from build123d import *

# Parameters (mm, degrees)
SKETCH040_W     = 20
SKETCH040_H     = 8
PAD021_DEPTH    = 10
POCKET019_DEPTH = 20
SKETCH042_R     = 1.5
POCKET020_DEPTH = 4
SKETCH043_W     = 4
SKETCH043_H     = 4.5
POCKET021_DEPTH = 5


with BuildPart() as part:
    # Sketch040 → Pad021 (new body)
    with BuildSketch(Plane.XY):
        Rectangle(SKETCH040_W, SKETCH040_H)
    extrude(amount=PAD021_DEPTH)

    # Sketch041 (on Face2 of Pad021) → Pocket019 (cut)
    with BuildSketch(Plane.YZ.offset(10)):
        Polygon((-4, 6.5), (-2.5, 10), (1, 10), (4, 6.5), (5, 6.5), (5, 11), (-5, 11), (-5, 6.5), align=None)
    extrude(amount=-POCKET019_DEPTH, mode=Mode.SUBTRACT)

    # Sketch042 (on Face8 of Pocket019) → Pocket020 (cut)
    with BuildSketch(Plane.XY.offset(10)):
        with Locations((-7.5, -0.75)):
            Circle(SKETCH042_R)
        with Locations((-2.5, -0.75)):
            Circle(SKETCH042_R)
        with Locations((2.5, -0.75)):
            Circle(SKETCH042_R)
        with Locations((7.5, -0.75)):
            Circle(SKETCH042_R)
    extrude(amount=-POCKET020_DEPTH, mode=Mode.SUBTRACT)

    # Sketch043 (on Face6 of Pocket020) → Pocket021 (cut)
    with BuildSketch(Plane.XZ.offset(4)):
        with Locations((-7.5, 3.25)):
            Rectangle(SKETCH043_W, SKETCH043_H)
        with Locations((-2.5, 3.25)):
            Rectangle(SKETCH043_W, SKETCH043_H)
        with Locations((2.5, 3.25)):
            Rectangle(SKETCH043_W, SKETCH043_H)
        with Locations((7.5, 3.25)):
            Rectangle(SKETCH043_W, SKETCH043_H)
    extrude(amount=-POCKET021_DEPTH, mode=Mode.SUBTRACT)


solid = part.part
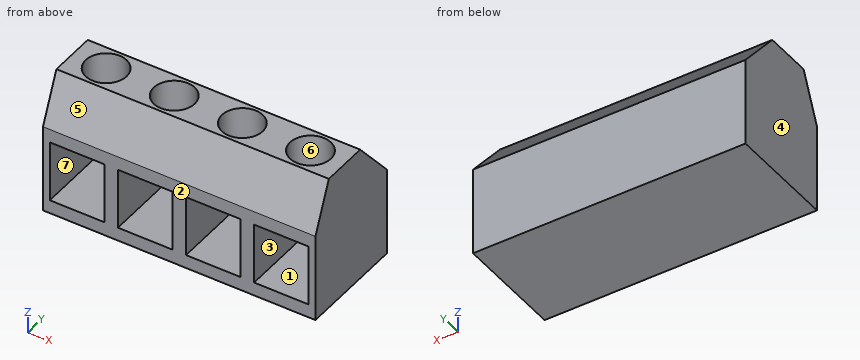
CAD build for the part. Positions are in the model's coordinates, mm. Face numbers are marked on the shaded views. A direction names the side the tool comes from. Give positions to 0.01 mm unless a question says otherwise; leave off trailing zeros. Loops run counter-clockwise (first coordinate to the right, second up) from the corner with the lowest first, then second, coordinate; pieces in that order, holes last. Notation, with made-up numbers: M 38.5,8.25 L 55.5,8.25 A16 cw 55.5,31.25 Z; hole C -19.75,22 d10. An arc over 180 degrees is marked long. Write each question's results on one line, items separated by ' | '.
Q1. Band-saw the part on C-C on y = -3. Write the cut outline in (x, z).
Geometry check:
outline: M -10,0 L 10,0 L 10,8.83 L -10,8.83 Z; hole M -9.5,1 L -5.5,1 L -5.5,5.5 L -9.5,5.5 Z; hole M -4.5,1 L -0.5,1 L -0.5,5.5 L -4.5,5.5 Z; hole M 0.5,1 L 4.5,1 L 4.5,5.5 L 0.5,5.5 Z; hole M 5.5,1 L 9.5,1 L 9.5,5.5 L 5.5,5.5 Z
Q2. Flat gauge pins, fed straight in: P1, Ø2, axis at x = 7, z = 8.5, coming from the +Y side; P2, Ø1.2, axis at x = -7, y = -0.5, coming from the +Z side; P3, Ø1.5, axis at x = 4.5, z = 8.5, coming from the -Y side. Where does each tip first touch, or does it go through?
Geometry check:
P1: stops at y = 3.14 | P2: stops at z = 6 | P3: stops at y = -3.46
Q3. Which spindle directions (+Z, -Z, +X, -X, +Y, -Y) get a long thin tool onto all of the face, cutting with end or side? Do the marked faces 5, 6 and 7. Say none if no direction does.
Geometry check:
face 5: +Z, +X, -X, -Y | face 6: +Z | face 7: -Y
Q4. Probe probe 1 along X at (y, z) = (0.5, 1.5); probe 2 along Z at (x, y) = (-3.75, -0.75); probe 3 along X at (y, z) = (-0.5, 8.25). List the from-to ranges inside material, lowest first.
Geometry check:
probe 1: x = -10 to -9.5, -5.5 to -4.5, -0.5 to 0.5, 4.5 to 5.5, 9.5 to 10 | probe 2: z = 0 to 1, 5.5 to 6 | probe 3: x = -10 to -8.98, -6.02 to -3.98, -1.02 to 1.02, 3.98 to 6.02, 8.98 to 10
Q5. Band-saw the part on A-A on z = 7. Write the cut outline in (x, y).
Geometry check:
outline: M -10,-3.79 L 10,-3.79 L 10,3.57 L -10,3.57 Z; hole C -7.5,-0.75 d3; hole C -2.5,-0.75 d3; hole C 2.5,-0.75 d3; hole C 7.5,-0.75 d3
Q6. Band-saw the part on D-D on x = 2.5. Write the cut outline in (y, z), and give its area (3 significant figures).
Geometry check:
outline: M -4,0 L 4,0 L 4,6.5 L 1,10 L 0.75,10 L 0.75,6 L -2.25,6 L -2.25,10 L -2.5,10 L -4,6.5 L -4,5.5 L 1,5.5 L 1,1 L -4,1 Z | area: 37.6 mm²
Q7. Band-saw the part on B-B on z = 4.5. Write the cut outline in (x, y).
Geometry check:
outline: M -10,-4 L -9.5,-4 L -9.5,1 L -5.5,1 L -5.5,-4 L -4.5,-4 L -4.5,1 L -0.5,1 L -0.5,-4 L 0.5,-4 L 0.5,1 L 4.5,1 L 4.5,-4 L 5.5,-4 L 5.5,1 L 9.5,1 L 9.5,-4 L 10,-4 L 10,4 L -10,4 Z
Q8. Mould opens along X. For the marked faces 1, 2, 3 and 4 say: pulls with the +X half, pulls with the -X half, needs draft (parallel to the pull), parting line crosses it, or undercut.
Geometry check:
face 1: undercut | face 2: needs draft | face 3: undercut | face 4: pulls with the -X half
